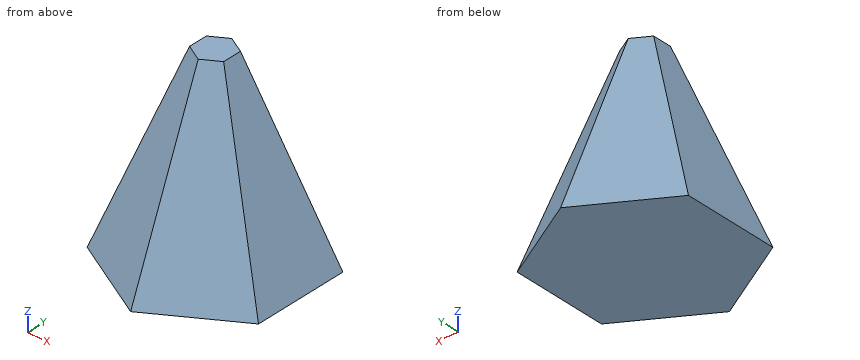
```python
from build123d import *

# Parameters (mm, degrees)
F1_DEPTH = 139.7
F1_TAPER = 20


with BuildPart() as f1:
    # F0 (on Top) → F1 (new body)
    with BuildSketch(Plane.XY):
        Polygon((63.5, -36.6617420935), (63.5, 36.6617420935), (0, 73.3234841871), (-63.5, 36.6617420935), (-63.5, -36.6617420935), (0, -73.3234841871), align=None)
    extrude(amount=F1_DEPTH, taper=F1_TAPER)


solid = f1.part
```
Build history of the part. All positions in model axes, mm. Coordinates: 2 decimals unless noted, no trailing zeros. Order: outer loops, then holes, each group sorted by start corner. A loop starts at its lowest first (then second) coordinate and runs counter-clockwise, first axis right, second up. Notation, with made-up numbers: (80, -1.5) -> (127, -1.5) arc R7 cw to (127, 4.5) -> close; hole circle Ø4 at (26, 16.25). An arc over 180 degrees is marked (long way). Answer in a Markdown table with one row per item. Add a question column.
Q1. Band-saw the part on A-A, the plane z = 120. List the corners of the cut face in (x, y), then the cut area to 3 significant figures.
Q2. Drop flat-ended pins along their axis: pin 1 (5 mm diameter, centred on y = -8, z = 41.5, fed in from -X); pin 2 (8 mm diameter, centred on y = 3, z = 114, fed in from -X); pin 3 (6 mm diameter, centred on x = 48, z = 22, fed in from +Y). Give the stop position or say it passes through.
Q3. Band-saw the part on C-C, the plane x = 41. List the corners of the cut face in (y, z), then the cut area to 3 significant figures.
Q4. Wall check: line 1 along Y through (x, z) = (14.5, 72); line 2 along X through (y, z) = (-55.5, 32); line 3 along Z through (x, y) = (-25.5, 27). Give the ranges that are in metal, low to high. Write a range as [from, to].
Q5. Band-saw the part on B-B, the plane y = 29. List the corners of the cut face in (x, z).
Q6. Band-saw the part on D-D, the plane z = 88.5. List the corners of the cut face in (x, y), then the cut area to 3 significant figures.
Answers follow:
| question | item | result |
|---|---|---|
| 1 | outline | (-19.82, -11.45) -> (0, -22.89) -> (19.82, -11.45) -> (19.82, 11.45) -> (0, 22.89) -> (-19.82, 11.45) -> close |
| 1 | area | 1,360 mm^2 |
| 2 | pin 1 | x = -49.31 |
| 2 | pin 2 | x = -23.46 |
| 2 | pin 3 | y = 38.51 |
| 3 | outline | (-49.65, 0) -> (49.65, 0) -> (23.67, 61.82) -> (-23.67, 61.82) -> close |
| 3 | area | 4,530 mm^2 |
| 4 | line 1 | [-34.69, 34.69] |
| 4 | line 2 | [-7.58, 7.58] |
| 4 | line 3 | [0, 75.19] |
| 5 | outline | (-63.5, 0) -> (63.5, 0) -> (50.23, 36.46) -> (0, 105.46) -> (-50.23, 36.46) -> close |
| 6 | outline | (-31.29, -18.06) -> (0, -36.13) -> (31.29, -18.06) -> (31.29, 18.06) -> (0, 36.13) -> (-31.29, 18.06) -> close |
| 6 | area | 3,390 mm^2 |
